Here's how the part is built. I have some questions about the finished solid (model axes, mm). A direction names the side the tool comes from. Round coordinates to 2 decimals unless told otherwise and drop trailing zeros. Loops run counter-clockwise (first coordinate to the right, second up) from the corner with the lowest first, then second, coordinate; pieces in that order, holes last. Notation, with made-up numbers: (62.25, 60.5) - (91.25, 60.5) arc R18 cw to (91.25, 67.5) - close; hole circle Ø9 at (27.5, 79). An arc over 180 degrees is marked (long way). Answer as a JSON object with one key per item and string values. Group by question number.
1) I want a section at A-A, the plane z = -87. Please give me the cut outline in (x, y), then the cut area to 3 significant figures.
2) Will these pins go through, and if not, where does the flat tip stop? P1, Ø7.5, axis at y = -104, z = -26.5, coming from the +X side; P2, Ø5, axis at x = 15.5, z = -30, coming from the +Y side; P3, Ø1.8, axis at x = -18, z = -75, coming from the -Y side; P4, Ø12, axis at y = -35, z = -15, coming from the -X side.
3) Which directions (+Z, -Z, +X, -X, +Y, -Y) give clear straight access to the entire face, cutting with the end or side of a thin tool? Please do faces 1 (the face through (0, -3, -40)), 2 (the face through (-11.72, -5.92, -88.84)), 3 (the face through (-0.04, -140.2, -2.85)), 4 (the face through (0, -133, -15)).
4) If I drill on line 1 along Z through (x, y) = (0, -5); line 2 along Z through (x, y) = (18, -7.75); line 3 along Z through (x, y) = (15, -9), over which ranges is the centre line in solid material (lowest first)? Write a range as [from, to].
5) I want a section at B-B, the plane y = -26.5. Please give me the cut outline in (x, z), then the cut area to 3 significant figures.
6) If we mould it in two halves opening along Y, with no side actions, what happens to faces 5 (the face through (0.056, -30.83, -19.416)), 6 (the face through (0, -101, -13)), 7 (the face through (-5.145, -141.477, -25.913)), 8 (the face through (6, -141, -15))? For each: pulls with the +Y half, pulls with the -Y half, needs draft (parallel to the pull), parting line crosses it, or undercut.
from build123d import *

# Parameters (mm, degrees)
Y_KSEKLIK_EKSTR_ZYON1_DEPTH = 40
IZIM2_W                     = 46
IZIM2_H                     = 18
Y_KSEKLIK_EKSTR_ZYON2_DEPTH = 70
IZIM3_W                     = 60
IZIM3_H                     = 6
KES_EKSTR_ZYON1_DEPTH       = 60
IZIM4_R                     = 4
IZIM4_R_2                   = 1.5
KES_EKSTR_ZYON2_DEPTH       = 60
Y_KSEKLIK_EKSTR_ZYON3_DEPTH = 46
PAH4_SIZE                   = 2.5
IZIM7_W                     = 5
IZIM7_H                     = 3
Y_KSEKLIK_EKSTR_ZYON4_DEPTH = 4
Y_KSEKLIK_EKSTR_ZYON5_DEPTH = 4
KES_EKSTR_ZYON4_DEPTH       = 10
RADYUS2_START               = -4
RADYUS2_DEPTH               = 8
RADYUS2_START_2             = -38.524937811
RADYUS2_2_DEPTH             = 35.524937811
RADYUS2_START_3             = -10
RADYUS2_3_DEPTH             = 20
Y_KSEKLIK_EKSTR_ZYON6_DEPTH = 8
IZIM12_W                    = 12
IZIM12_H                    = 24
Y_KSEKLIK_EKSTR_ZYON7_DEPTH = 5
RADYUS3_R                   = 3
IZIM13_R                    = 1.5
KES_EKSTR_ZYON5_DEPTH       = 35


with BuildPart() as part:
    # Çizim1 → Yükseklik-Ekstrüzyon1 (new body)
    with BuildSketch(Plane.XY):
        with BuildLine():
            Line((-8, 0), (-23, 0))
            Line((-23, 0), (-23, -18))
            Line((-23, -18), (23, -18))
            Line((23, -18), (23, 0))
            Line((23, 0), (8, 0))
            ThreePointArc((8, 0), (0, -8), (-8, 0))
        make_face()
    extrude(amount=-Y_KSEKLIK_EKSTR_ZYON1_DEPTH)

    # Çizim2 → Yükseklik-Ekstrüzyon2 (add)
    with BuildSketch(Plane(origin=(0, 0, -40), x_dir=(-1, 0, 0), z_dir=(0, 0, -1))):
        with Locations((0, -9)):
            Rectangle(IZIM2_W, IZIM2_H)
    extrude(amount=Y_KSEKLIK_EKSTR_ZYON2_DEPTH)

    # Çizim3 → Kes-Ekstrüzyon1 (cut)
    with BuildSketch(Plane(origin=(23, 0, 0), x_dir=(0, 0, -1), z_dir=(1, 0, 0))):
        with Locations((80, -15)):
            Rectangle(IZIM3_W, IZIM3_H)
    extrude(amount=-KES_EKSTR_ZYON1_DEPTH, mode=Mode.SUBTRACT)

    # Çizim4 → Kes-Ekstrüzyon2 (cut)
    with BuildSketch(Plane(origin=(0, 0, 0), x_dir=(1, 0, 0), z_dir=(0, 1, 0))):
        with Locations(Location((0, 75, 0), (0, 0, 180))):
            Circle(IZIM4_R)
        with Locations(Location((0, 57, 0), (0, 0, 180))):
            Circle(IZIM4_R_2)
        with Locations(Location((-18, 75, 0), (0, 0, 180))):
            Circle(IZIM4_R_2)
        with Locations(Location((0, 93, 0), (0, 0, 180))):
            Circle(IZIM4_R_2)
        with Locations(Location((18, 75, 0), (0, 0, 180))):
            Circle(IZIM4_R_2)
        with BuildLine():
            Line((-15.202795796, 92.324116139), (-8.131727984, 85.253048327))
            ThreePointArc((-8.131727984, 85.253048327), (-8.131727984, 83.131727984), (-10.253048327, 83.131727984))
            Line((-10.253048327, 83.131727984), (-17.324116139, 90.202795796))
            ThreePointArc((-17.324116139, 90.202795796), (-17.324116139, 92.324116139), (-15.202795796, 92.324116139))
        make_face()
        with BuildLine():
            Line((15.202795796, 92.324116139), (8.131727984, 85.253048327))
            ThreePointArc((8.131727984, 85.253048327), (8.131727984, 83.131727984), (10.253048327, 83.131727984))
            Line((10.253048327, 83.131727984), (17.324116139, 90.202795796))
            ThreePointArc((17.324116139, 90.202795796), (17.324116139, 92.324116139), (15.202795796, 92.324116139))
        make_face()
        with BuildLine():
            Line((17.324116139, 59.797204204), (10.253048327, 66.868272016))
            ThreePointArc((10.253048327, 66.868272016), (8.131727984, 66.868272016), (8.131727984, 64.746951673))
            Line((8.131727984, 64.746951673), (15.202795796, 57.675883861))
            ThreePointArc((15.202795796, 57.675883861), (17.324116139, 57.675883861), (17.324116139, 59.797204204))
        make_face()
        with BuildLine():
            Line((-15.202795796, 57.675883861), (-8.131727984, 64.746951673))
            ThreePointArc((-8.131727984, 64.746951673), (-8.131727984, 66.868272016), (-10.253048327, 66.868272016))
            Line((-10.253048327, 66.868272016), (-17.324116139, 59.797204204))
            ThreePointArc((-17.324116139, 59.797204204), (-17.324116139, 57.675883861), (-15.202795796, 57.675883861))
        make_face()
    extrude(amount=-KES_EKSTR_ZYON2_DEPTH, mode=Mode.SUBTRACT)

    # Çizim5 → Yükseklik-Ekstrüzyon3 (add)
    with BuildSketch(Plane(origin=(23, 0, 0), x_dir=(0, 0, -1), z_dir=(1, 0, 0))):
        Polygon((110, 0), (110, 8), (100, 8), (100, 3), (104, 3), (104, 0), align=None)
    extrude(amount=-Y_KSEKLIK_EKSTR_ZYON3_DEPTH)

    # Pah4
    pah4_edges = [part.edges().sort_by_distance(p)[0] for p in [
        (23, 8, -105),
        (0, 8, -110),
        (-23, 8, -105),
        (23, -2, -110),
        (-23, -2, -110),
        (0, -12, -110),
        (-23, -18, -25),
        (-23, -15, -50),
        (23, -18, -25),
        (-23, -12, -80),
        (0, -18, -50),
        (23, -15, -50),
        (23, -12, -80),
    ]]
    chamfer(pah4_edges, length=PAH4_SIZE)

    # Çizim7 → Yükseklik-Ekstrüzyon4 (add)
    with BuildSketch(Plane.XY.offset(-104)):
        with Locations((-20.5, 1.5)):
            Rectangle(IZIM7_W, IZIM7_H)
        with Locations((20.5, 1.5)):
            Rectangle(IZIM7_W, IZIM7_H)
    extrude(amount=Y_KSEKLIK_EKSTR_ZYON4_DEPTH)

    # Çizim9 → Yükseklik-Ekstrüzyon5 (add, symmetric)
    with BuildSketch(Plane(origin=(0, 0, 0), x_dir=(0, 0, -1), z_dir=(1, 0, 0))):
        Polygon((8, -18), (34, -18), (22, -138), (8, -138), align=None)
    extrude(amount=Y_KSEKLIK_EKSTR_ZYON5_DEPTH, both=True)

    # Çizim10 → Kes-Ekstrüzyon4 (cut)
    with BuildSketch(Plane(origin=(4, 0, 0), x_dir=(0, 0, -1), z_dir=(1, 0, 0))):
        Polygon((13, -132.742033617), (13, -133), (17.475062189, -133), (18.000954253, -127.741079364), (13.707106781, -132.034926836), align=None)
        Polygon((13, -122.42585543), (13, -129.913606492), (16.743875531, -126.169730961), align=None)
        Polygon((14.414213562, -121.011641868), (18.286653963, -124.884082268), (19.147196274, -116.278659157), align=None)
        Polygon((13, -109.817193202), (13, -119.597428306), (17.890117552, -114.707310754), align=None)
        Polygon((14.414213562, -108.40297964), (19.432895983, -113.421662061), (20.548158744, -102.269034459), align=None)
        Polygon((13, -94.406606035), (13, -106.988766077), (19.291080021, -100.697686056), align=None)
        Polygon((14.414213562, -92.992392472), (20.833858453, -99.412037363), (22.260446207, -85.146159828), align=None)
        Polygon((13, -75.571443941), (13, -91.57817891), (21.003367485, -83.574811425), align=None)
        Polygon((14.414213562, -74.157230378), (22.546145916, -82.289162732), (24.353241995, -64.218201946), align=None)
        Polygon((13, -52.55069027), (13, -72.743016816), (23.096163273, -62.646853543), align=None)
        Polygon((14.414213562, -51.136476708), (24.638941704, -61.36120485), (26.911103514, -38.639586757), align=None)
        Polygon((13, -24.414213562), (13, -49.722263146), (25.654024792, -37.068238354), align=None)
        Polygon((14.414213562, -23), (27.196803223, -35.782589661), (28.475062189, -23), align=None)
    extrude(amount=-KES_EKSTR_ZYON4_DEPTH, mode=Mode.SUBTRACT)

    # Radyus2: read off the stored shape, not the designer's step
    # Radyus2 outline → Radyus2 (add)
    with BuildSketch(Plane.YZ.offset(RADYUS2_START)):
        with BuildLine():
            Line((-18, -38.524937811), (-18, -34))
            Line((-18, -34), (-22.502481405, -33.54975186))
            ThreePointArc((-22.502481405, -33.54975186), (-19.292737332, -35.169911207), (-18, -38.524937811))
        make_face()
        with BuildLine():
            ThreePointArc((-18, -3), (-19.464466094, -6.535533906), (-23, -8))
            Line((-23, -8), (-18, -8))
            Line((-18, -8), (-18, -3))
        make_face()
    extrude(amount=RADYUS2_DEPTH)

    # Radyus2 2 outline → Radyus2 2 (add)
    with BuildSketch(Plane.XY.offset(RADYUS2_START_2)):
        with BuildLine():
            Line((4, -18), (4, -23))
            ThreePointArc((4, -23), (5.464466094, -19.464466094), (9, -18))
            Line((9, -18), (4, -18))
        make_face()
        with BuildLine():
            Line((-4, -23), (-4, -18))
            Line((-4, -18), (-9, -18))
            ThreePointArc((-9, -18), (-5.464466094, -19.464466094), (-4, -23))
        make_face()
    extrude(amount=RADYUS2_2_DEPTH)

    # Radyus2 3 outline → Radyus2 3 (cut)
    with BuildSketch(Plane.YZ.offset(RADYUS2_START_3)):
        with BuildLine():
            Line((-22.502481405, -33.54975186), (-23, -33.5))
            Line((-23, -33.5), (-23, -38.524937811))
            Line((-23, -38.524937811), (-18, -38.524937811))
            ThreePointArc((-18, -38.524937811), (-19.292737332, -35.169911207), (-22.502481405, -33.54975186))
        make_face()
        with BuildLine():
            Line((-23, -3), (-23, -8))
            ThreePointArc((-23, -8), (-19.464466094, -6.535533906), (-18, -3))
            Line((-18, -3), (-23, -3))
        make_face()
    extrude(amount=RADYUS2_3_DEPTH, mode=Mode.SUBTRACT)

    # Çizim11 → Yükseklik-Ekstrüzyon6 (add)
    with BuildSketch(Plane.ZY.offset(4)):
        Polygon((-22, -138), (-21.927011625, -138.729883751), (-8, -138), align=None)
    extrude(amount=-Y_KSEKLIK_EKSTR_ZYON6_DEPTH)

    # Çizim12 → Yükseklik-Ekstrüzyon7 (add)
    with BuildSketch(Plane(origin=(0, -137.203896927, 7.190551547), x_dir=(1, 0, 0), z_dir=(0, -0.9986295347545744, 0.05233595624293665))):
        with Locations((0, -22.184460391)):
            Rectangle(IZIM12_W, IZIM12_H)
    extrude(amount=Y_KSEKLIK_EKSTR_ZYON7_DEPTH)

    # Radyus3
    radyus3_edges = [part.edges().sort_by_distance(p)[0] for p in [
        (6, -141.489547187, -26.816220339),
        (6, -140.233484238, -2.849111505),
        (-6, -140.233484238, -2.849111505),
        (-6, -141.489547187, -26.816220339),
    ]]
    fillet(radyus3_edges, radius=RADYUS3_R)

    # Çizim13 → Kes-Ekstrüzyon5 (cut)
    with BuildSketch(Plane(origin=(0, 0, 0), x_dir=(1, 0, 0), z_dir=(0, 1, 0))):
        with Locations(Location((-15.5, 10, 0), (0, 0, 270))):
            Circle(IZIM13_R)
        with Locations(Location((-15.5, 30, 0), (0, 0, 270))):
            Circle(IZIM13_R)
        with Locations(Location((15.5, 30, 0), (0, 0, 90))):
            Circle(IZIM13_R)
        with Locations(Location((15.5, 10, 0), (0, 0, 90))):
            Circle(IZIM13_R)
    extrude(amount=-KES_EKSTR_ZYON5_DEPTH, mode=Mode.SUBTRACT)


solid = part.part
Outcome:
{
 "1": {"outline": "(-23, -9.5) - (-20.5, -12) - (-14.12, -12) - (-14.12, 0) - (-23, 0) - close; (-9.88, -12) - (9.88, -12) - (9.88, 0) - (-9.88, 0) - close; (14.12, -12) - (20.5, -12) - (23, -9.5) - (23, 0) - (14.12, 0) - close", "area": "444 mm^2"},
 "2": {"P1": "x = 4", "P2": "y = 0", "P3": "through", "P4": "x = -4"},
 "3": {"face 1": "+Z, +Y", "face 2": "+Y, -Y", "face 3": "+Z, +X, -X", "face 4": "+X, -X"},
 "4": {"line 1": "[-110, -94.5], [-91.5, -79], [-71, -58.5], [-55.5, -40]", "line 2": "[-110, -76.5], [-73.5, 0]", "line 3": "[-110, -92.12], [-87.88, -62.12], [-57.88, -31.41], [-28.59, -11.41], [-8.59, 0]"},
 "5": {"outline": "(-4, -33.15) - (4, -33.15) - (4, -28.13) - (-4, -28.13) - close; (-4, -17.91) - (4, -17.91) - (4, -15.09) - (-4, -15.09) - close; (-4, -13) - (4, -13) - (4, -8) - (-4, -8) - close", "area": "103 mm^2"},
 "6": {"face 5": "undercut", "face 6": "undercut", "face 7": "pulls with the -Y half", "face 8": "needs draft"}
}
